Geometry: final body of the model. Coordinates: model frame, mm. A direction names the side the tool comes from. Coordinates: 2 decimals unless noted, no trailing zeros. Order: outer loops, then holes, each group sorted by start corner. A loop starts at its lowest first (then second) coordinate and runs counter-clockwise, first axis right, second up. Notation, with made-up numbers: M -37.75,-16 L -30.75,-16 A18 ccw -30.75,-3 Z; hole C 66,-9.75 d5. An arc over 180 degrees is marked long. Write item = value, one per line.
from build123d import *

# Parameters (mm, degrees)
SKETCH1_R           = 1.5875
BOSS_EXTRUDE1_DEPTH = 4.7625


with BuildPart() as part:
    # Sketch1 → Boss-Extrude1 (new body)
    with BuildSketch(Plane.XY):
        Polygon((0, 0), (12.7, 0), (12.7, -4.7625), (19.05, -4.7625), (19.05, 31.75), (-6.35, 31.75), (-6.35, -4.7625), (0, -4.7625), align=None)
        with Locations(Location((6.35, 19.05, 0), (0, 0, 180))):
            Circle(SKETCH1_R, mode=Mode.SUBTRACT)
        with Locations(Location((6.35, 26.67, 0), (0, 0, 180))):
            Circle(SKETCH1_R, mode=Mode.SUBTRACT)
        with Locations(Location((13.97, 19.05, 0), (0, 0, 180))):
            Circle(SKETCH1_R, mode=Mode.SUBTRACT)
        with Locations(Location((-1.27, 19.05, 0), (0, 0, 180))):
            Circle(SKETCH1_R, mode=Mode.SUBTRACT)
        with Locations(Location((6.35, 11.43, 0), (0, 0, 180))):
            Circle(SKETCH1_R, mode=Mode.SUBTRACT)
    extrude(amount=BOSS_EXTRUDE1_DEPTH)


solid = part.part
1) Line query: L1, parallel to X at y = 19.05, z = 3.05; L2, parallel to Y at x = 6.35, z = 3.45; L3, parallel to X at y = 11.43, z = 2.05. Output: solid intervals per line, ascending.
Numbers:
L1 = -6.35 to -2.86, 0.32 to 4.76, 7.94 to 12.38, 15.56 to 19.05
L2 = 0 to 9.84, 13.02 to 17.46, 20.64 to 25.08, 28.26 to 31.75
L3 = -6.35 to 4.76, 7.94 to 19.05
2) Set-up query: faces 5 (the face through (12.7, -2, 2)), 6 (the face through (16, -4.762, 2)). Return all of +Z, -Z, +X, -X, +Y, -Y with unobstructed straight access to the full face (end or side cutting, diameter ignored); none if empty.
Numbers:
face_5 = +Z, -Z, -Y
face_6 = +Z, -Z, +X, -X, -Y
3) Section A-A, the plane x = 6.35. Return loops of the section in (y, z).
Numbers:
outline = M 0,0 L 9.84,0 L 9.84,4.76 L 0,4.76 Z; M 13.02,0 L 17.46,0 L 17.46,4.76 L 13.02,4.76 Z; M 20.64,0 L 25.08,0 L 25.08,4.76 L 20.64,4.76 Z; M 28.26,0 L 31.75,0 L 31.75,4.76 L 28.26,4.76 Z
4) Pin query (flat end, axial travel): pin 1 (1.4 mm diameter, centred on x = 5, z = 2, fed in from -Y). Return the tip coordinate at first contact, or that it passes through.
Numbers:
pin_1 = 0
5) Section C-C, the plane y = 11.43. Return loops of the section in (x, z), and give its area (3 significant figures).
Numbers:
outline = M -6.35,0 L 4.76,0 L 4.76,4.76 L -6.35,4.76 Z; M 7.94,0 L 19.05,0 L 19.05,4.76 L 7.94,4.76 Z
area = 106 mm²
6) Mould query, pull axis X, two halves, no side actions, for faces 1 (the face through (6.69, 28.22, 2.35)), 2 (the face through (5.5, 17.71, 2.35)), 3 (the face through (-3, -4.762, 2)), 4 (the face through (-6.35, 14, 2)). Classes: pulls with the +X half, pulls with the -X half, needs draft (parallel to the pull), parting line crosses it, or undercut.
Numbers:
face_1 = undercut
face_2 = undercut
face_3 = needs draft
face_4 = pulls with the -X half
7) Section B-B, the plane x = -1.27. Return loops of the section in (y, z).
Numbers:
outline = M -4.76,0 L 17.46,0 L 17.46,4.76 L -4.76,4.76 Z; M 20.64,0 L 31.75,0 L 31.75,4.76 L 20.64,4.76 Z
8) Section D-D, the plane z = 1.4. Give the number of separate pieces and of enclosed holes in the cut face, and give its area (3 significant figures).
Numbers:
separate_pieces = 1
enclosed_holes = 5
area = 827 mm²
